Check sheet for the drawn part. Datum: minimum x, y, z corner. Units: mm. A direction names the side the tool comes from. Round coordinates to 2 decimals unless told otherwise and drop trailing zeros. Loops run counter-clockwise (first coordinate to the right, second up) from the corner with the lowest first, then second, coordinate; pieces in that order, holes last.
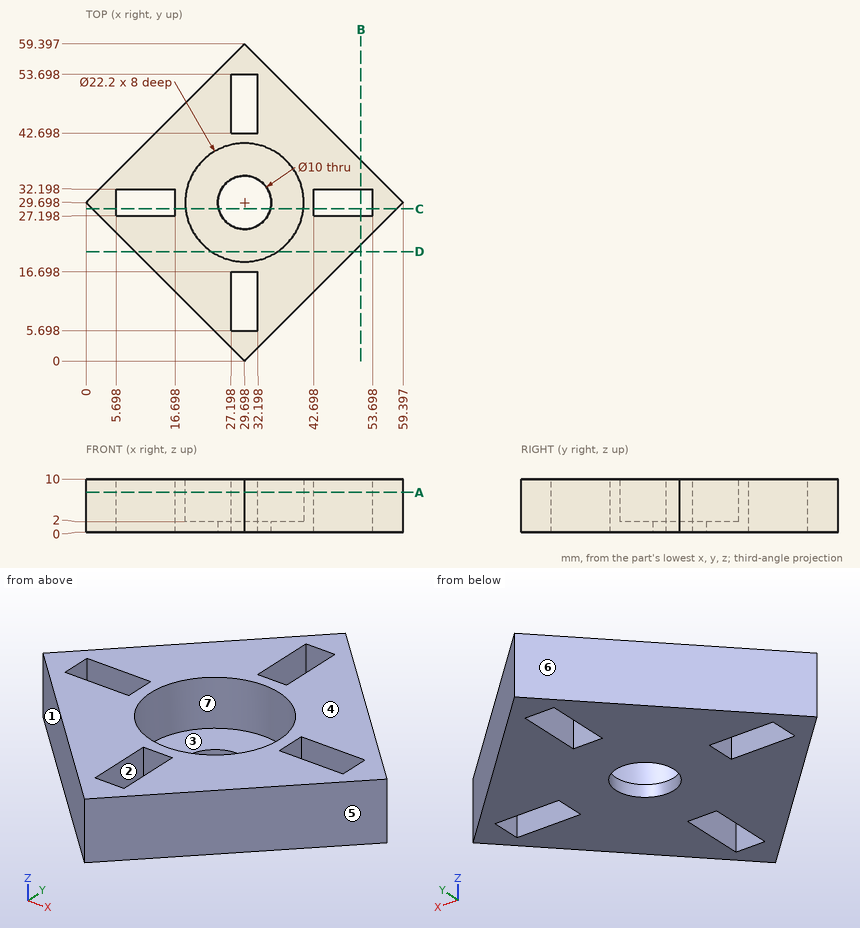
1) Sectioned sample at A-A, the plane z = 7.5. Record the cut outline in (x, y).
Report:
outline: (0, 29.7) - (29.7, 0) - (59.4, 29.7) - (29.7, 59.4) - close; hole (5.7, 27.2) - (16.7, 27.2) - (16.7, 32.2) - (5.7, 32.2) - close; hole circle Ø22.2 at (29.7, 29.7); hole (27.2, 5.7) - (32.2, 5.7) - (32.2, 16.7) - (27.2, 16.7) - close; hole (27.2, 42.7) - (32.2, 42.7) - (32.2, 53.7) - (27.2, 53.7) - close; hole (42.7, 27.2) - (53.7, 27.2) - (53.7, 32.2) - (42.7, 32.2) - close
2) Access from +Z, -Z, +X, -X, +Y, -Y to the whole of each face (thin tool, end or side, straight path). Record for the marked faces 1, 2 and 3.
Report:
face 1: +Z, -Z, -X, -Y
face 2: +Z, -Z
face 3: +Z
3) Sectioned sample at D-D, the plane y = 20.5. Record the cut outline in (x, z) (1 decimal).
Report:
outline: (9.2, 0) - (50.2, 0) - (50.2, 10) - (35.9, 10) - (35.9, 2) - (23.5, 2) - (23.5, 10) - (9.2, 10) - close
4) Sectioned sample at C-C, the plane y = 28.5. Record the cut outline in (x, z) (1 decimal).
Report:
outline: (1.2, 0) - (5.7, 0) - (5.7, 10) - (1.2, 10) - close; (16.7, 0) - (24.8, 0) - (24.8, 2) - (18.7, 2) - (18.7, 10) - (16.7, 10) - close; (34.6, 0) - (42.7, 0) - (42.7, 10) - (40.7, 10) - (40.7, 2) - (34.6, 2) - close; (53.7, 0) - (58.2, 0) - (58.2, 10) - (53.7, 10) - close
5) Sectioned sample at B-B, the plane x = 51.5. Record the cut outline in (y, z) (1 decimal), then the cut area to 3 significant figures.
Report:
outline: (21.8, 0) - (27.2, 0) - (27.2, 10) - (21.8, 10) - close; (32.2, 0) - (37.6, 0) - (37.6, 10) - (32.2, 10) - close
area: 108 mm2
6) Scan lines: line 1 along Y through (x, z) = (30, 5.75) (1 decimal); line 2 along Y through (x, z) = (30, 0.5) (1 decimal); line 3 along Z through (x, y) = (34, 32.5). Record each from-to range of solid material in increasing order.
Report:
line 1: y = 0.3 to 5.7, 16.7 to 18.6, 40.8 to 42.7, 53.7 to 59.1
line 2: y = 0.3 to 5.7, 16.7 to 24.7, 34.7 to 42.7, 53.7 to 59.1
line 3: z = 0 to 2
7) Mould release check, pull along X, two halves, no side actions. Record for the marked faces 4, 5, 6 and 7: +X half, -X half, draft (parallel to the pull), parting line (faces both ways), or undercut.
Report:
face 4: draft
face 5: +X half
face 6: -X half
face 7: undercut
8) Gauge pin test, flat ends, axial feed: pin 1 (11 mm diameter, centred on x = 32.5, y = 30, fed in from +Z); pin 2 (5.5 mm diameter, centred on y = 29, z = 7, fed in from +X); pin 3 (1.5 mm diameter, centred on y = 9, z = 5, fed in from +X). Record the tip position at first contact, or that the pin passes through.
Report:
pin 1: stops at z = 2
pin 2: stops at x = 59.4
pin 3: stops at x = 39.45
